Check sheet for the modelled part. Datum: model origin and axes. Units: mm. Face numbers are marked on the shaded views. Coordinates: 2 decimals unless noted, no trailing zeros. Write each loop counter-clockwise with the first axis right and the second up, starting at its lowest first coordinate (ties: lowest second). Pieces come first, ordered by that corner, then holes. Notation, with made-up numbers: M 31.5,27.5 L 88.5,27.5 A24 ccw 88.5,46.5 Z; hole C 20.5,23 d4. An arc over 180 degrees is marked long. Answer as CSV lines item,"result". Start each with the question number.
1) Section check D-D (y = 16.75). Record the cut outline in (x, z), and give its area (3 significant figures).
2) Draft check along X on the marked faces 1, 2 and 3. Enter one of: +X half, -X half, draft (parallel to the pull), parting line (faces both ways), or undercut.
3) Section check A-A (z = 0). Record the cut outline in (x, y), and give its area (3 significant figures).
4) Material ranges on L1, parallel to Z at x = 0, y = 16.5; L2, parallel to X at y = 22, z = 1; L3, parallel to X at y = 24, z = -20.5, recorded low to high. Write a range as [from, to].
5) Section check B-B (x = 0). Record the cut outline in (y, z).
6) Section check C-C (y = 10.5). Record the cut outline in (x, z), and give its area (3 significant figures).
7) Go/stop test with flat-tipped pins: pin 1 Ø1.5 at (x, z) = (25.5, -46) entering from +Y; pin 2 Ø2 at (y, z) = (21, 25.5) entering from -X; pin 3 Ø1 at (x, y) = (-37, 4.5) entering from -Z. Record where each tip stops, or that it passes through.
from build123d import *

# Parameters (mm, degrees)
ESQUISSE1_R             = 57.5
ESQUISSE1_R_2           = 47.5
BOSS_EXTRU_3_DEPTH      = 30
ENL_V_MAT_EXTRU_4_DEPTH = 15
ENL_V_MAT_EXTRU_5_DEPTH = 15
ENL_V_MAT_EXTRU_6_DEPTH = 15
ENL_V_MAT_EXTRU_7_DEPTH = 15
ESQUISSE10_R            = 2.776949087
ESQUISSE10_R_2          = 2.5
ENL_V_MAT_EXTRU_8_DEPTH = 10


with BuildPart() as part:
    # Esquisse1 → Boss.-Extru.3 (new body)
    with BuildSketch(Plane(origin=(0, 0, 0), x_dir=(1, 0, 0), z_dir=(0, 1, 0))):
        with Locations(Location((0, 0, 0), (0, 0, 270))):
            Circle(ESQUISSE1_R)
        with Locations(Location((0, 0, 0), (0, 0, 270))):
            Circle(ESQUISSE1_R_2, mode=Mode.SUBTRACT)
    extrude(amount=BOSS_EXTRU_3_DEPTH)

    # Esquisse4 → Enlèv. mat.-Extru.4 (cut)
    with BuildSketch(Plane(origin=(0, 0, 0), x_dir=(-1, 0, 0), z_dir=(0, -1, 0))):
        Polygon((-4.740706844, -47.262836337), (-14.579980258, -45.207014673), (-17.999133934, -61.771502914), (-8.15986052, -63.827324578), align=None)
    extrude(amount=-ENL_V_MAT_EXTRU_4_DEPTH, mode=Mode.SUBTRACT)

    # Esquisse6 → Enlèv. mat.-Extru.5 (cut)
    with BuildSketch(Plane(origin=(0, 0, 0), x_dir=(-1, 0, 0), z_dir=(0, -1, 0))):
        Polygon((37.97805027, -11.470285743), (58.779258548, -16.171123772), (59.719426153, -6.534405813), (38.918217876, -1.833567784), align=None)
    extrude(amount=-ENL_V_MAT_EXTRU_5_DEPTH, mode=Mode.SUBTRACT)

    # Esquisse7 → Enlèv. mat.-Extru.6 (cut)
    with BuildSketch(Plane(origin=(0, 0, 0), x_dir=(-1, 0, 0), z_dir=(0, -1, 0))):
        Polygon((10.091528645, 41.476841185), (15.939537835, 59.219106356), (6.91972705, 60.755447754), (1.071717859, 43.013182582), align=None)
    extrude(amount=-ENL_V_MAT_EXTRU_6_DEPTH, mode=Mode.SUBTRACT)

    # Esquisse8 → Enlèv. mat.-Extru.7 (cut)
    with BuildSketch(Plane(origin=(0, 0, 0), x_dir=(-1, 0, 0), z_dir=(0, -1, 0))):
        Polygon((-42.754189526, 0.991012316), (-70.16329298, 5.019646945), (-68.868374707, 16.242271981), (-41.459271253, 12.213637353), align=None)
    extrude(amount=-ENL_V_MAT_EXTRU_7_DEPTH, mode=Mode.SUBTRACT)

    # Esquisse10 → Enlèv. mat.-Extru.8 (cut)
    with BuildSketch(Plane(origin=(0, 30, 0), x_dir=(1, 0, 0), z_dir=(0, 1, 0))):
        with Locations(Location((45.289109306, -26.55459618, 0), (0, 0, 270))):
            Circle(ESQUISSE10_R)
        with Locations(Location((26.55459618, 45.289109306, 0), (0, 0, 270))):
            Circle(ESQUISSE10_R_2)
        with Locations(Location((-26.55459618, -45.289109306, 0), (0, 0, 270))):
            Circle(ESQUISSE10_R_2)
        with Locations(Location((-45.289109306, 26.55459618, 0), (0, 0, 270))):
            Circle(ESQUISSE10_R_2)
    extrude(amount=-ENL_V_MAT_EXTRU_8_DEPTH, mode=Mode.SUBTRACT)


solid = part.part
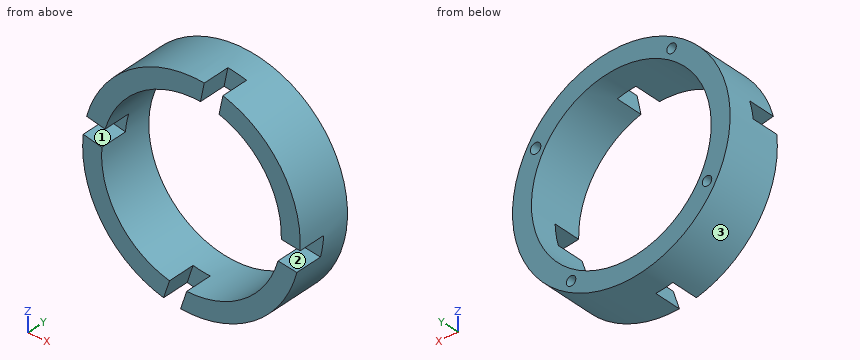
Results found:
1,outline,"C 0,0 d115; hole C 0,0 d95"
1,area,"3,300 mm2"
2,face 1,"undercut"
2,face 2,"+X half"
2,face 3,"parting line"
3,outline,"M -57.5,0 L -47.5,0 L -47.5,30 L -57.5,30 Z; M 47.5,0 L 57.5,0 L 57.5,30 L 47.5,30 Z"
3,area,"600 mm2"
4,L1,"z = [-57.5, -47.5], [47.5, 57.5]"
4,L2,"x = [-57.49, -47.49], [47.49, 57.49]"
4,L3,"x = [-53.72, -42.85], [42.85, 53.72]"
5,outline,"M 0,-57.5 L 30,-57.5 L 30,-47.5 L 0,-47.5 Z; M 0,47.5 L 30,47.5 L 30,57.5 L 0,57.5 Z"
6,outline,"M -57.19,5.96 A57.5 ccw -14.74,-55.58 L -11.6,-46.06 A47.5 cw -47.35,3.74 Z; M -55.4,15.41 L -45.63,13.2 A47.5 cw 4.74,47.26 L 6.77,57.1 A57.5 ccw Z; M -5.75,-57.21 A57.5 ccw 55.69,-14.31 L 45.73,-12.84 A47.5 cw -2.53,-47.43 Z; M 14.58,45.21 A47.5 cw 47.47,-1.68 L 57.41,-3.15 A57.5 ccw 16.61,55.05 Z"
6,area,"2,900 mm2"
7,pin 1,"stops at y = 20"
7,pin 2,"stops at x = -52.02"
7,pin 3,"stops at z = -44.43"
